Model file for the job. Use its own axes, mm. A direction names the side the tool comes from. Give positions to 0.01 mm unless a question says otherwise; leave off trailing zeros. Loops run counter-clockwise (first coordinate to the right, second up) from the corner with the lowest first, then second, coordinate; pieces in that order, holes last. Notation, with made-up numbers: M -6,1.5 L 21,1.5 A21 ccw 21,36.5 Z; hole C 48.5,22.5 d11. An arc over 180 degrees is marked long. Answer in a Markdown table with one row per item.
```python
from build123d import *

# Parameters (mm, degrees)
SKETCH_R     = 15
SKETCH_R_2   = 7.5
SKETCH_R_3   = 2
PAD_DEPTH    = 9
SKETCH001_R  = 2.03355
POCKET_DEPTH = 38.000995
CHAMFER_SIZE = 1


with BuildPart() as part:
    # Sketch → Pad (new body)
    with BuildSketch(Plane.XY):
        with BuildLine():
            ThreePointArc((18.999995, 0.014309), (-0.007154, 18.999999), (-19, 0))
            Line((-19, -75), (-19, 0))
            Line((-15, -75), (-19, -75))
            Line((-15, -75), (-15, -50))
            Line((-15, -50), (15, -50))
            Line((15, -50), (15, -75))
            Line((18.999995, -75), (15, -75))
            Line((18.999995, 0.014309), (18.999995, -75))
        make_face()
        Circle(SKETCH_R, mode=Mode.SUBTRACT)
        with Locations((0, -32)):
            Circle(SKETCH_R_2, mode=Mode.SUBTRACT)
        with Locations((-11.162674, -20.837326)):
            Circle(SKETCH_R_3, mode=Mode.SUBTRACT)
        with Locations((11.162674, -20.837326)):
            Circle(SKETCH_R_3, mode=Mode.SUBTRACT)
        with Locations((-11.162674, -43.162674)):
            Circle(SKETCH_R_3, mode=Mode.SUBTRACT)
        with Locations((11.162674, -43.162674)):
            Circle(SKETCH_R_3, mode=Mode.SUBTRACT)
    extrude(amount=PAD_DEPTH)

    # Sketch001 (on Face5 of Pad) → Pocket (cut, through all)
    with BuildSketch(Plane.YZ.offset(18.999995)):
        with Locations((-63, 4.5)):
            Circle(SKETCH001_R)
    extrude(amount=-POCKET_DEPTH, mode=Mode.SUBTRACT)

    # Chamfer
    chamfer_edges = [part.edges().sort_by_distance(p)[0] for p in [
        (-15, 0, 9),
    ]]
    chamfer(chamfer_edges, length=CHAMFER_SIZE)


solid = part.part
```
Q1. Saw through at B-B (y = -67.5). Give the cut face in (x, z), and give its area (3 significant figures).
Reported:
| item | result |
|---|---|
| outline | M -19,0 L -15,0 L -15,9 L -19,9 Z; M 15,0 L 19,0 L 19,9 L 15,9 Z |
| area | 72.0 mm² |
Q2. Saw through at D-D (y = -32). Give the cut face in (x, z).
Reported:
| item | result |
|---|---|
| outline | M -19,0 L -7.5,0 L -7.5,9 L -19,9 Z; M 7.5,0 L 19,0 L 19,9 L 7.5,9 Z |
Q3. Probe probe 1 along Y at (x, z) = (0.5, 1.25); probe 2 along X at (y, z) = (-58, 4.75); probe 3 along Z at (x, y) = (-17, -63). List the from-to ranges inside material, lowest first.
Reported:
| item | result |
|---|---|
| probe 1 | -50 to -39.48, -24.52 to -14.99, 14.99 to 18.99 |
| probe 2 | -19 to -15, 15 to 19 |
| probe 3 | 0 to 2.47, 6.53 to 9 |
Q4. 3-axis set-ups, long thin cutter, end or side, ignore diameter. For faces 1 (the face through (-10.087, -41.476, 4.437)), 2 (the face through (15, -62, 2)): which of +Z, -Z, +X, -X, +Y, -Y reach the whole face in a straight line?
Reported:
| item | result |
|---|---|
| face 1 | +Z, -Z |
| face 2 | +Z, -Z, -Y |
Q5. Saw through at A-A (x = 0). Give the cut face in (y, z), and give its area (3 significant figures).
Reported:
| item | result |
|---|---|
| outline | M -50,0 L -39.5,0 L -39.5,9 L -50,9 Z; M -24.5,0 L -15,0 L -15,8 L -16,9 L -24.5,9 Z; M 15,0 L 19,0 L 19,9 L 16,9 L 15,8 Z |
| area | 215 mm² |
Q6. Drop flat-ended pins along their axis: pin 1 (2 mm diameter, centred on x = -12.5, z = 4, fed in from -Y); pin 2 (2 mm diameter, centred on x = 1, z = 4, fed in from +Y). Give the stop position or say it passes through.
Reported:
| item | result |
|---|---|
| pin 1 | y = -50 |
| pin 2 | y = 19 |
Q7. Saw through at C-C (z = 4.5). Give the number of separate pieces and of enclosed holes in the cut face, and give its area (3 significant figures).
Reported:
| item | result |
|---|---|
| separate pieces | 3 |
| enclosed holes | 6 |
| area | 1,700 mm² |
Q8. Mould opens along Y. For faces 3 (the face through (10.73, -22.79, 4.44)), 4 (the face through (-10.24, -22.61, 4.44)), 5 (the face through (8, -27, 9)), 6 (the face through (-17, -75, 4)) say: released by +Y, released by -Y, zero draft, split by the parting line, or undercut.
Reported:
| item | result |
|---|---|
| face 3 | undercut |
| face 4 | undercut |
| face 5 | zero draft |
| face 6 | released by -Y |
